Autodesk Inventor part; units mm, degrees
ref_plane "YZ Plane" through (0, 0, 0) normal (1, 0, 0) x (0, 1, 0)
ref_plane "XZ Plane" through (0, 0, 0) normal (0, 1, 0) x (-1, 0, 0)
ref_plane "XY Plane" through (0, 0, 0) normal (0, 0, 1) x (1, 0, 0)
sketch "Sketch1" plane through (0, 0, 0) normal (0, 1, 0) x (-1, 0, 0)
  line L0 (-38, 30) -> (38, 30)
  line L1 (38, 30) -> (38, -30)
  line L2 (38, -30) -> (-38, -30)
  line L3 (-38, -30) -> (-38, 30)
  line L4 (-38, 30) -> (38, -30) construction
  line L5 (38, 30) -> (-38, -30) construction
  point P0 (0, 0)
  dimension "d0" = 60
  dimension "d1" = 76
extrude "Extrusion1" add sketch "Sketch1" along normal blind 26
sketch "Sketch2" plane through (-38, 0, 30) normal (0, 0, 1) x (1, 0, 0)
  line L0 (0, 0) -> (0, 26)
  line L1 (76, 0) -> (76, 26)
  line L2 (0, 23) -> (76, 23)
  line L3 (76, 23) -> (76, 3)
  line L4 (76, 3) -> (0, 3)
  line L5 (0, 3) -> (0, 23)
  line L6 (0, 26) -> (76, 26)
  line L7 (0, 0) -> (76, 0)
  point P0 (38, 0)
  point P1 (0, 3)
  dimension "d4" = 3
  dimension "d5" = 3
extrude "Extrusion2" cut sketch "Sketch2" against normal blind 20 contours L0 L2 L1 L4
sketch "Sketch3" plane through (0, 26, 0) normal (0, 1, 0) x (1, 0, 0)
  arc A0 (15.9974, 14) -> (-16, 13.7099) centre (-0.0026, 14) ccw
  line L0 (38, 30) -> (-38, 30)
  line L1 (-38, 30) -> (-38, -30)
  arc A1 (-38, -7) -> (-16, 13.7099) centre (-54.3067, 32.3627) ccw
  line L2 (38, -30) -> (38, 30)
  line L3 (38, 30) -> (-38, 30)
  line L4 (38, -30) -> (-38, -30)
  arc A2 (15.9974, 14) -> (38, -7) centre (54.478, 32.2913) ccw
  line L5 (-38, -10) -> (-38, -30)
  line L6 (-38, -7) -> (38, -7)
  line L7 (38, -10) -> (-38, -10)
  point P0 (0, 0)
  point P1 (38, -7)
  point P2 (-0.0026, 30)
  dimension "d8" = 32
  dimension "d10" = 3
extrude "Extrusion3" cut sketch "Sketch3" against normal through all contours A0 L0 L2 A2 | A0 A1 L1 L0
sketch "Sketch5" plane through (0, 26, 0) normal (0, 1, 0) x (1, 0, 0)
  arc A0 (15.9974, 14) -> (-16, 13.7099) centre (-0.0026, 14) ccw
  line L0 (38, 30) -> (-38, 30)
  line L1 (-38, 30) -> (-38, -30)
  arc A1 (-38, -7) -> (-16, 13.7099) centre (-54.3067, 32.3627) ccw
  line L2 (38, -30) -> (38, 30)
  line L3 (38, 30) -> (-38, 30)
  line L4 (38, -30) -> (-38, -30)
  arc A2 (15.9974, 14) -> (38, -7) centre (54.478, 32.2913) ccw
  line L5 (-38, -10) -> (-38, -30)
  line L6 (-38, -7) -> (38, -7)
  line L7 (38, -10) -> (-38, -10)
  point P0 (0, 0)
  point P1 (0, 0)
  point P2 (38, -7)
  point P3 (-0.0026, 30)
  dimension "d13" = 32
  dimension "d14" = 3
sketch "Sketch7" plane through (0, 0, 0) normal (0, -1, 0) x (1, 0, 0)
  arc A0 (-16, -13.7099) -> (15.9974, -14) centre (-0.0026, -14) ccw
  arc A1 (-16, -13.7099) -> (15.9974, -14) centre (-0.0026, -14) ccw
  line L0 (38, 30) -> (38, 7)
  arc A2 (38, 7) -> (15.9974, -14) centre (54.478, -32.2913) ccw
  arc A3 (-16, -13.7099) -> (-38, 7) centre (-54.3067, -32.3627) ccw
  arc A4 (-16, -13.7099) -> (-38, 7) centre (-54.3067, -32.3627) ccw
  line L1 (-38, 10) -> (38, 10)
  line L2 (38, 10) -> (-38, 10)
  line L3 (38, 7) -> (38, 10)
  line L4 (-38, 7) -> (-38, 30)
  line L5 (-38, 7) -> (-38, 10)
  arc A5 (38, 7) -> (15.9974, -14) centre (54.478, -32.2913) ccw
  line L6 (38, 7) -> (-38, 7)
  point P0 (0, 0)
extrude "Extrusion4" cut sketch "Sketch5" against normal blind 4.875 contours A2 L6 A1 A0
extrude "Extrusion5" cut sketch "Sketch7" against normal blind 4.875 contours A3 L6 A2 A0
sketch "Sketch9" plane through (0, 21.125, 0) normal (0, 1, 0) x (1, 0, 0)
  arc A0 (15.9974, 14) -> (-16, 13.7099) centre (-0.0026, 14) ccw
  line L0 (3.6635, 20.35) -> (7.3297, 14)
  line L1 (7.3297, 14) -> (3.6635, 7.65)
  line L2 (3.6635, 7.65) -> (-3.6688, 7.65)
  line L3 (-3.6688, 7.65) -> (-7.335, 14)
  line L4 (-7.335, 14) -> (-3.6688, 20.35)
  line L5 (-3.6688, 20.35) -> (3.6635, 20.35)
  point P0 (0, 0)
  dimension "d19" = 12.7
extrude "Extrusion6" cut sketch "Sketch9" against normal through all
sketch "Sketch10" plane through (0, 26, 0) normal (0, 1, 0) x (1, 0, 0)
  circle A0 centre (0, -20) radius 5.8489
  circle A1 centre (25, -20) radius 5.871
  circle A2 centre (-25, -20) radius 5.8765
  line L0 (-38, -7) -> (-38, -30)
  line L1 (-38, -30) -> (38, -30)
  point P0 (0, 0)
  dimension "d23" = 10
  dimension "d24" = 10
  dimension "d25" = 10
  dimension "d27" = 0
  dimension "d28" = 25
  dimension "d29" = 25
hole "Hole1" at (-25, 26, 20) at (0, 26, 20) at (25, 26, 20) direction (0, -1, 0) diameter 5.5 end through all
properties part number "CH-1-02-BearingBracket"
Geometry check sheet. Reference: the model listing, model coordinates, mm. A direction names the side the tool comes from. Give positions to 0.01 mm unless a question says otherwise; leave off trailing zeros. Loops run counter-clockwise (first coordinate to the right, second up) from the corner with the lowest first, then second, coordinate; pieces in that order, holes last. Notation, with made-up numbers: (-15.5, -7.75) -> (23.5, -7.75) arc R22 ccw to (23.5, 11.25) -> close; hole circle Ø5 at (61.25, 37). An arc over 180 degrees is marked (long way). Answer in a Markdown table with one row per item. Add a question column.
1) Cross-section at C-C on x = 0. Record the boundary of the cut face in (y, z) (3 decimals), and give its area (3 significant figures).
2) Cross-section at D-D on x = 25. Record the boundary of the cut face in (y, z) (3 decimals).
3) Draft check along X on faces 1 (the face through (0, 13, -30)), 2 (the face through (24.879, 1.479, 17.253)), 3 (the face through (-38, 14, 9)). Enter one of: pulls with the +X half, pulls with the -X half, needs draft (parallel to the pull), parting line crosses it, or undercut.
4) Material ranges on probe 1 along X at (y, z) = (2.15, 20); probe 2 along Y at (x, z) = (-16.5, 18); probe 3 along Z at (x, y) = (0, 1.3), recorded low to high. Write a range as from..to.
5) Gauge pin test, flat ends, axial feed: P1, Ø4.5, axis at x = -25, z = 20, coming from the +Y side; P2, Ø4, axis at x = 28.5, y = 6, coming from the -Z side; P3, Ø2, axis at x = 6, z = -9.5, coming from the -Y side (3 decimals); P4, Ø1, axis at x = -10, z = -9, coming from the +Y side (3 decimals). Record the tip position at first contact, or that the pin passes through.
6) Set-up check for faces 4 (the face through (-1, 4.875, -7)), 5 (the face through (1, 1, 30)), 6 (the face through (-1, 24, 7)), 7 (the face through (24.904, 13.114, -1.62)), 8 (the face through (0, 13, -20.35)): record each of +Z, -Z, +X, -X, +Y, -Y from which the full face is reachable in a straight line by a thin tool's end or side.
7) Cross-section at A-A on z = 20. State how many separate pieces and enclosed holes the cut face has, and give its area (3 significant figures).
Outcome:
| question | item | result |
|---|---|---|
| 1 | outline | (0, 7) -> (4.875, 7) -> (4.875, -7.65) -> (21.125, -7.65) -> (21.125, 7) -> (26, 7) -> (26, 17.25) -> (23, 17.25) -> (23, 10) -> (3, 10) -> (3, 17.25) -> (0, 17.25) -> close; (0, 22.75) -> (3, 22.75) -> (3, 30) -> (0, 30) -> close; (4.875, -30) -> (21.125, -30) -> (21.125, -20.35) -> (4.875, -20.35) -> close; (23, 22.75) -> (26, 22.75) -> (26, 30) -> (23, 30) -> close |
| 1 | area | 560 mm^2 |
| 2 | outline | (0, 7) -> (4.875, 7) -> (4.875, -1.528) -> (21.125, -1.528) -> (21.125, 7) -> (26, 7) -> (26, 17.25) -> (23, 17.25) -> (23, 10) -> (3, 10) -> (3, 17.25) -> (0, 17.25) -> close; (0, 22.75) -> (3, 22.75) -> (3, 30) -> (0, 30) -> close; (23, 22.75) -> (26, 22.75) -> (26, 30) -> (23, 30) -> close |
| 3 | face 1 | parting line crosses it |
| 3 | face 2 | undercut |
| 3 | face 3 | pulls with the -X half |
| 4 | probe 1 | x = -38..-27.75, -22.25..-2.75, 2.75..22.25, 27.75..38 |
| 4 | probe 2 | y = 0..3, 23..26 |
| 4 | probe 3 | z = 7..17.25, 22.75..30 |
| 5 | P1 | passes through |
| 5 | P2 | stops at z = -0.16 |
| 5 | P3 | stops at y = 4.875 |
| 5 | P4 | stops at y = 21.125 |
| 6 | face 4 | -Z, +X, -X, -Y |
| 6 | face 5 | +Z, +X, -X, +Y, -Y |
| 6 | face 6 | -Z, +X, -X, +Y |
| 6 | face 7 | -Z, +X, +Y, -Y |
| 6 | face 8 | +Y, -Y |
| 7 | separate pieces | 8 |
| 7 | enclosed holes | 0 |
| 7 | area | 357 mm^2 |
